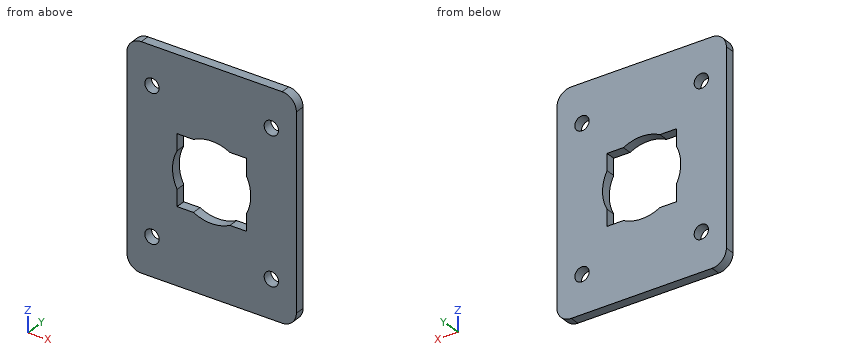
from build123d import *

# Parameters (mm, degrees)
SKETCH_1_W          = 35.5
SKETCH_1_H          = 46
EXTRUDE_1_DEPTH     = 2
FILLET_2_R          = 3
SKETCH_3_R          = 1.5
CUT_EXTRUDE_1_DEPTH = 10


with BuildPart() as part:
    # 草图1 → 凸台-拉伸1 (new body)
    with BuildSketch(Plane(origin=(0, 0, 0), x_dir=(1, 0, 0), z_dir=(0, 1, 0))):
        with Locations((0.862287952, 7.25)):
            Rectangle(SKETCH_1_W, SKETCH_1_H)
        with BuildLine():
            Line((-6.387712048, 3.418877449), (-6.387712048, 0))
            Line((-6.387712048, 0), (-2.968834599, 0))
            ThreePointArc((-2.968834599, 0), (0.862287952, -0.95), (4.693410503, 0))
            Line((4.693410503, 0), (8.112287952, 0))
            Line((8.112287952, 0), (8.112287952, 3.418877449))
            ThreePointArc((8.112287952, 3.418877449), (9.062287952, 7.25), (8.112287952, 11.081122551))
            Line((8.112287952, 11.081122551), (8.112287952, 14.5))
            Line((8.112287952, 14.5), (4.693410503, 14.5))
            ThreePointArc((4.693410503, 14.5), (0.862287952, 15.45), (-2.968834599, 14.5))
            Line((-2.968834599, 14.5), (-6.387712048, 14.5))
            Line((-6.387712048, 14.5), (-6.387712048, 11.081122551))
            ThreePointArc((-6.387712048, 11.081122551), (-7.337712048, 7.25), (-6.387712048, 3.418877449))
        make_face(mode=Mode.SUBTRACT)
    extrude(amount=EXTRUDE_1_DEPTH)

    # 圆角2
    fillet_2_edges = [part.edges().sort_by_distance(p)[0] for p in [
        (-16.887712048, 1, -30.25),
        (18.612287952, 1, -30.25),
        (18.612287952, 1, 15.75),
        (-16.887712048, 1, 15.75),
    ]]
    fillet(fillet_2_edges, radius=FILLET_2_R)

    # 草图3 → 切除-拉伸1 (cut)
    with BuildSketch(Plane.XZ):
        with Locations(Location((-11.637712048, 7.75, 0), (0, 0, 270))):
            Circle(SKETCH_3_R)
        with Locations(Location((-11.637712048, -22.25, 0), (0, 0, 270))):
            Circle(SKETCH_3_R)
        with Locations(Location((13.362287952, -22.25, 0), (0, 0, 270))):
            Circle(SKETCH_3_R)
        with Locations(Location((13.362287952, 7.75, 0), (0, 0, 270))):
            Circle(SKETCH_3_R)
    extrude(amount=-CUT_EXTRUDE_1_DEPTH, mode=Mode.SUBTRACT)


solid = part.part
Check sheet for the modelled part. Datum: model origin and axes. Units: mm. Round coordinates to 2 decimals unless told otherwise and drop trailing zeros. Order: outer loops, then holes, each group sorted by start corner. A loop starts at its lowest first (then second) coordinate and runs counter-clockwise, first axis right, second up. Notation, with made-up numbers: M 18.25,-8 L 52.25,-8 A16 ccw 52.25,19 Z; hole C -1,-0.75 d10. An arc over 180 degrees is marked long. One line per item, written item: value. Start each with the question number.
1. Section check C-C on y = 1.5. Enter the section's corners in (x, z), and give its area (3 significant figures).
2. Gauge pin test, flat end, axial feed: P1, Ø2.5, axis at x = -11.64, z = -22.25, coming from the -Y side. Record the tip position at first contact, or that the pin passes through.
3. Section check A-A on z = 7.75. Enter the section's corners in (x, y).
4. Scan lines: line 1 along X through (y, z) = (0.8, 7.75); line 2 along Z through (x, y) = (7.5, 1.05); line 3 along Z through (x, y) = (0.5, 1.55). Record each from-to range of solid material in increasing order.
5. Section check B-B on z = -5.5. Enter the section's corners in (x, y), and give its area (3 significant figures).
Results found:
1. outline: M -16.89,-27.25 A3 ccw -13.89,-30.25 L 15.61,-30.25 A3 ccw 18.61,-27.25 L 18.61,12.75 A3 ccw 15.61,15.75 L -13.89,15.75 A3 ccw -16.89,12.75 Z; hole C -11.64,-22.25 d3; hole C -11.64,7.75 d3; hole M -6.39,-14.5 L -2.97,-14.5 A8.2 ccw 4.69,-14.5 L 8.11,-14.5 L 8.11,-11.08 A8.2 ccw 8.11,-3.42 L 8.11,0 L 4.69,0 A8.2 ccw -2.97,0 L -6.39,0 L -6.39,-3.42 A8.2 ccw -6.39,-11.08 Z; hole C 13.36,-22.25 d3; hole C 13.36,7.75 d3
1. area: 1,370 mm^2
2. P1: through
3. outline: M -16.89,0 L -13.14,0 L -13.14,2 L -16.89,2 Z; M -10.14,0 L 11.86,0 L 11.86,2 L -10.14,2 Z; M 14.86,0 L 18.61,0 L 18.61,2 L 14.86,2 Z
4. line 1: -16.89 to -13.14, -10.14 to 11.86, 14.86 to 18.61
4. line 2: -30.25 to -14.5, 0 to 15.75
4. line 3: -30.25 to -15.44, 0.94 to 15.75
5. outline: M -16.89,0 L -7.15,0 L -7.15,2 L -16.89,2 Z; M 8.87,0 L 18.61,0 L 18.61,2 L 8.87,2 Z
5. area: 39.0 mm^2
